Check sheet for the drawn part. Datum: minimum x, y, z corner. Units: mm. Give positions to 0.01 mm unless a question says otherwise; leave off trailing zeros. Loops run counter-clockwise (first coordinate to the right, second up) from the corner with the lowest first, then second, coordinate; pieces in that order, holes last. Notation, with made-up numbers: (31, 87.25) - (71, 87.25) arc R12 cw to (71, 106.25) - close; hole circle Ø9 at (89, 88.25). An arc over 180 degrees is marked (long way). Use a Markdown table: item, result. Add a question column.
1. Cross-section at B-B on y = 57.5. Enter the section's corners in (x, z), and give its area (3 significant figures).
2. Cross-section at A-A on x = 1.5. Enter the section's corners in (y, z).
3. Depth check by flat-ended pin: P1, Ø1.5, axis at x = 2, z = 2, coming from the +Y side; P2, Ø12, axis at x = 12.5, y = 57.5, coming from the -Z side; P3, Ø0.9, axis at y = 8.5, z = 1.5, coming from the -X side; P4, Ø0.9, axis at y = 24.5, z = 1, coming from the -X side. Enter the tip coordinate at first touch or a pass-through.
4. Cross-section at D-D on x = 18. Enter the section's corners in (y, z).
5. Material ranges on L1, parallel to Y at x = 1, z = 1.6; L2, parallel to Y at x = 12, z = 2; L3, parallel to Y at x = 7.25, z = 0.25, recorded low to high.
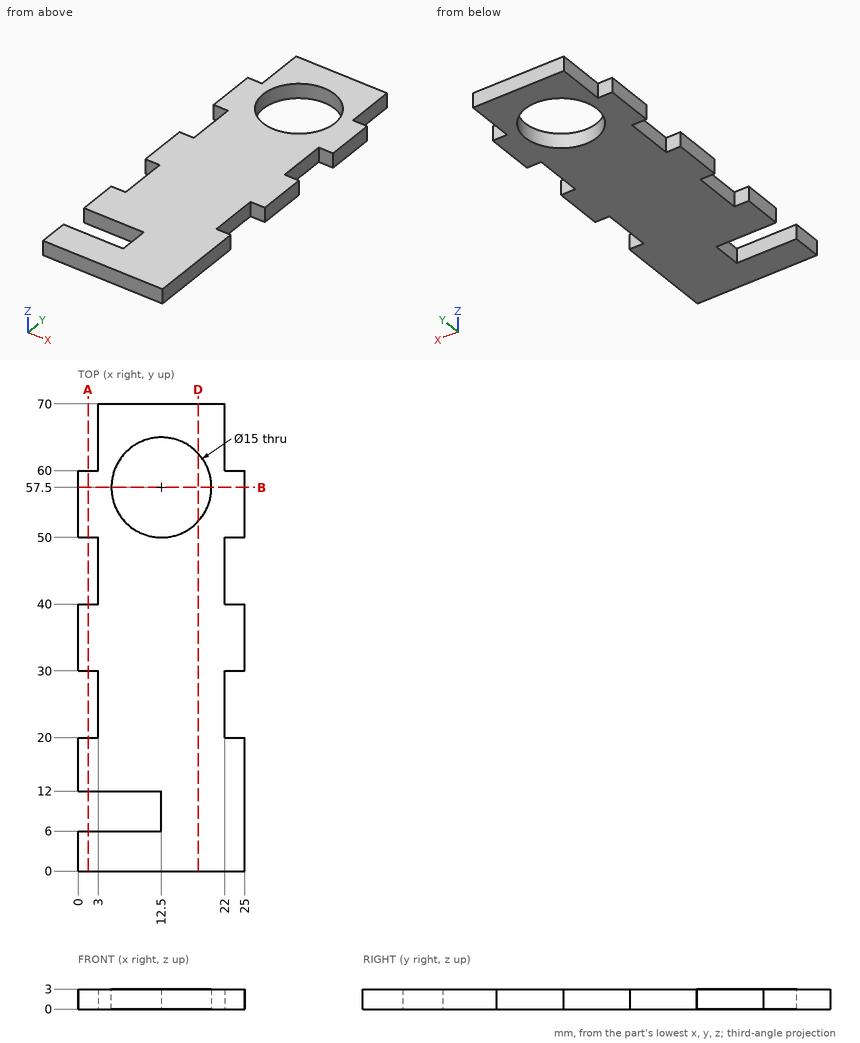
Values found:
| question | item | result |
|---|---|---|
| 1 | outline | (0, 0) - (5, 0) - (5, 3) - (0, 3) - close; (20, 0) - (25, 0) - (25, 3) - (20, 3) - close |
| 1 | area | 30.0 mm2 |
| 2 | outline | (0, 0) - (6, 0) - (6, 3) - (0, 3) - close; (12, 0) - (20, 0) - (20, 3) - (12, 3) - close; (30, 0) - (40, 0) - (40, 3) - (30, 3) - close; (50, 0) - (60, 0) - (60, 3) - (50, 3) - close |
| 3 | P1 | stops at y = 60 |
| 3 | P2 | passes through |
| 3 | P3 | stops at x = 12.5 |
| 3 | P4 | stops at x = 3 |
| 4 | outline | (0, 0) - (52.4, 0) - (52.4, 3) - (0, 3) - close; (62.6, 0) - (70, 0) - (70, 3) - (62.6, 3) - close |
| 5 | L1 | y = 0 to 6, 12 to 20, 30 to 40, 50 to 60 |
| 5 | L2 | y = 0 to 6, 12 to 50.02, 64.98 to 70 |
| 5 | L3 | y = 0 to 6, 12 to 52.14, 62.86 to 70 |
